The figure shows three views and two pictorial views of one solid part (mm, origin at its lowest corner). Answer the questions. Coordinates: 2 decimals unless noted, no trailing zeros. Order: outer loops, then holes, each group sorted by start corner. A loop starts at its lowest first (then second) coordinate and runs counter-clockwise, first axis right, second up. Notation, with made-up numbers: (38.5, -38.5) -> (56.5, -38.5) arc R13 ccw to (56.5, -15.5) -> close; hole circle Ø11 at (42, 68.25). An arc over 180 degrees is marked (long way). Return JSON: item names as keys, results as strings.
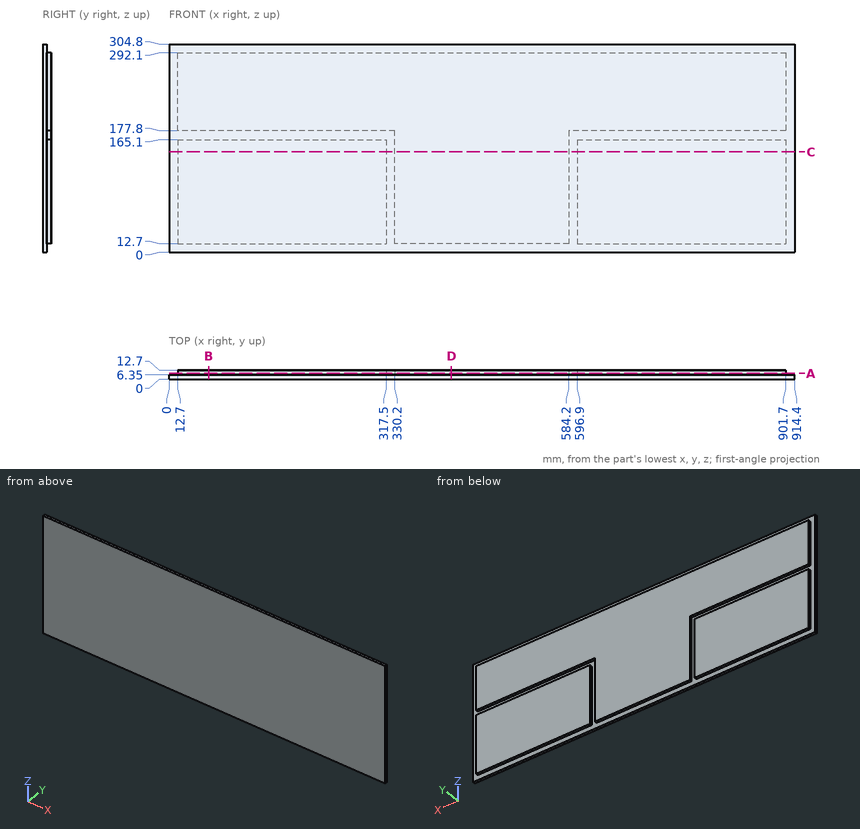
1. Each of these flat-tipped pins is pushed along its axis until it touches: pin 1 Ø7 at (y, z) = (10, 92) entering from -X; pin 2 Ø5 at (x, y) = (771, 10.5) entering from -Z; pin 3 Ø1.9 at (x, y) = (583.5, 8.5) entering from +Z. Where does it stop, or does it pass through?
Answer block:
{"pin 1": "stops at x = 12.7", "pin 2": "stops at z = 12.7", "pin 3": "stops at z = 292.1"}
2. The part is cut by section B-B on x = 57.5. Give the vertices of the cut face in (y, z).
Answer block:
{"outline": "(0, 0) -> (6.35, 0) -> (6.35, 12.7) -> (12.7, 12.7) -> (12.7, 165.1) -> (6.35, 165.1) -> (6.35, 177.8) -> (12.7, 177.8) -> (12.7, 292.1) -> (6.35, 292.1) -> (6.35, 304.8) -> (0, 304.8) -> close"}
3. Consider line 1 (X direction, y = 12.25, z = 116); line 2 (Z direction, x = 99, y = 9.5); line 3 (X direction, y = 12, z = 245.5). Determine where each line is inside the solid, lowest interval first. Write a range as from..to.
Answer block:
{"line 1": "x = 12.7..317.5, 330.2..584.2, 596.9..901.7", "line 2": "z = 12.7..165.1, 177.8..292.1", "line 3": "x = 12.7..901.7"}
4. The part is cut by section C-C on z = 147. Give the vertices of the cut face in (x, y), and give its area (3 significant figures).
Answer block:
{"outline": "(0, 0) -> (914.4, 0) -> (914.4, 6.35) -> (901.7, 6.35) -> (901.7, 12.7) -> (596.9, 12.7) -> (596.9, 6.35) -> (584.2, 6.35) -> (584.2, 12.7) -> (330.2, 12.7) -> (330.2, 6.35) -> (317.5, 6.35) -> (317.5, 12.7) -> (12.7, 12.7) -> (12.7, 6.35) -> (0, 6.35) -> close", "area": "11,300 mm2"}
5. The part is cut by section A-A on y = 8.5. Give the vertices of the cut face in (x, z), and give its area (3 significant figures).
Answer block:
{"outline": "(12.7, 12.7) -> (317.5, 12.7) -> (317.5, 165.1) -> (12.7, 165.1) -> close; (12.7, 177.8) -> (330.2, 177.8) -> (330.2, 12.7) -> (584.2, 12.7) -> (584.2, 177.8) -> (901.7, 177.8) -> (901.7, 292.1) -> (12.7, 292.1) -> close; (596.9, 12.7) -> (901.7, 12.7) -> (901.7, 165.1) -> (596.9, 165.1) -> close", "area": "236,000 mm2"}
6. The part is cut by section D-D on x = 412.5. Give the vertices of the cut face in (y, z), and give its area (3 significant figures).
Answer block:
{"outline": "(0, 0) -> (6.35, 0) -> (6.35, 12.7) -> (12.7, 12.7) -> (12.7, 292.1) -> (6.35, 292.1) -> (6.35, 304.8) -> (0, 304.8) -> close", "area": "3,710 mm2"}
